```python
from build123d import *

# Parameters (mm, degrees)
BOSS_EXTRUDE2_DEPTH = 3
SKETCH2_W           = 44
SKETCH2_H           = 70
BOSS_EXTRUDE3_DEPTH = 10
BOSS_EXTRUDE4_DEPTH = 3
CUT_EXTRUDE1_REACH  = 103.047
SKETCH7_R           = 2.5


with BuildPart() as part:
    # Sketch1 → Boss-Extrude2 (new body)
    with BuildSketch(Plane.XY):
        with BuildLine():
            Line((-11.286595542, 0), (32.713404458, 0))
            Line((32.713404458, 0), (32.713404458, 49))
            Line((32.713404458, 49), (34.849610431, 49))
            Line((34.849610431, 49), (34.849610431, 64))
            Line((34.849610431, 64), (24.849610431, 64))
            Line((24.849610431, 64), (19.349610431, 45.378267854))
            Line((19.349610431, 45.378267854), (19.349610431, 40.378267854))
            ThreePointArc((19.349610431, 40.378267854), (9.849610431, 30.878267854), (0.349610431, 40.378267854))
            Line((0.349610431, 40.378267854), (0.349610431, 45.378267854))
            Line((0.349610431, 45.378267854), (-3.422801515, 64))
            Line((-3.422801515, 64), (-13.422801515, 64))
            Line((-13.422801515, 64), (-13.422801515, 49))
            Line((-13.422801515, 49), (-11.286595542, 49))
            Line((-11.286595542, 49), (-11.286595542, 0))
        make_face()
    extrude(amount=BOSS_EXTRUDE2_DEPTH)

    # Sketch2 → Boss-Extrude3 (add)
    with BuildSketch(Plane(origin=(0, 0, 0), x_dir=(1, 0, 0), z_dir=(0, 1, 0))):
        with Locations((10.713404458, 35)):
            Rectangle(SKETCH2_W, SKETCH2_H)
    extrude(amount=BOSS_EXTRUDE3_DEPTH)

    # Sketch4 → Boss-Extrude4 (add)
    with BuildSketch(Plane.XY.offset(-70)):
        with BuildLine():
            Line((34.849610431, 64), (24.849610431, 64))
            Line((24.849610431, 64), (19.349610431, 45.378267854))
            Line((19.349610431, 45.378267854), (19.349610431, 40.378267854))
            ThreePointArc((19.349610431, 40.378267854), (9.849610431, 30.878267854), (0.349610431, 40.378267854))
            Line((0.349610431, 40.378267854), (0.349610431, 45.378267854))
            Line((0.349610431, 45.378267854), (-3.422801515, 64))
            Line((-3.422801515, 64), (-13.422801515, 64))
            Line((-13.422801515, 64), (-13.422801515, 49))
            Line((-13.422801515, 49), (-11.286595542, 49))
            Line((-11.286595542, 49), (-11.286595542, 0))
            Line((-11.286595542, 0), (32.713404458, 0))
            Line((32.713404458, 0), (32.713404458, 49))
            Line((32.713404458, 49), (34.849610431, 49))
            Line((34.849610431, 49), (34.849610431, 64))
        make_face()
    extrude(amount=BOSS_EXTRUDE4_DEPTH)

    # Sketch7 → Cut-Extrude1 (cut, up to next)
    with BuildSketch(Plane(origin=(0, 0, 0), x_dir=(1, 0, 0), z_dir=(0, 1, 0)), mode=Mode.PRIVATE) as cut_extrude1_sk1:
        with Locations(Location((10.713404458, 48.5, 0), (0, 0, 270))):
            Circle(SKETCH7_R)
    cut_extrude1_tool1 = extrude(cut_extrude1_sk1.sketch, amount=CUT_EXTRUDE1_REACH, mode=Mode.PRIVATE) & part.part
    # Sketch7 → Cut-Extrude1 (cut, up to next)
    with BuildSketch(Plane(origin=(0, 0, 0), x_dir=(1, 0, 0), z_dir=(0, 1, 0)), mode=Mode.PRIVATE) as cut_extrude1_sk2:
        with Locations(Location((10.713404458, 18.5, 0), (0, 0, 270))):
            Circle(SKETCH7_R)
    cut_extrude1_tool2 = extrude(cut_extrude1_sk2.sketch, amount=CUT_EXTRUDE1_REACH, mode=Mode.PRIVATE) & part.part
    add(cut_extrude1_tool1.solids().sort_by_distance((10.713404, 0, -48.5))[0], mode=Mode.SUBTRACT)
    add(cut_extrude1_tool2.solids().sort_by_distance((10.713404, 0, -18.5))[0], mode=Mode.SUBTRACT)


solid = part.part
```
The model under review builds one solid part; all positions refer to its coordinate system, in mm. A direction names the side the tool comes from. Round coordinates to 2 decimals unless told otherwise and drop trailing zeros. Loops run counter-clockwise (first coordinate to the right, second up) from the corner with the lowest first, then second, coordinate; pieces in that order, holes last. Notation, with made-up numbers: (-21.75, 1.25) -> (-5.75, 1.25) arc R18 cw to (-5.75, 22.25) -> close; hole circle Ø4 at (36.25, -5.5). An arc over 180 degrees is marked (long way). Answer in a Markdown table with one row per item.
1) Consider section D-D, the plane x = 1.5. Write out the cut boundary in (y, z).
Taken from the geometry:
| item | result |
|---|---|
| outline | (0, -70) -> (35.85, -70) -> (35.85, -67) -> (10, -67) -> (10, 0) -> (35.85, 0) -> (35.85, 3) -> (0, 3) -> close |
2) For pin 1 Ø2.5 at (y, z) = (43, 1.5) entering from +X; pin 2 Ø1.1 at (x, z) = (34, 2) entering from -Y; pin 3 Ø13 at (x, z) = (-0.5, -33.5) entering from +Y; pin 4 Ø6 at (x, z) = (30, -53) entering from -Y, all flat-tipped, find the tip position at first contact; note any pin that passes through.
Taken from the geometry:
| item | result |
|---|---|
| pin 1 | stops at x = 32.71 |
| pin 2 | stops at y = 49 |
| pin 3 | stops at y = 10 |
| pin 4 | stops at y = 0 |
3) Draft analysis for pull direction X (two halves, no side actions). For faces 1 (the flat face through (0.35, 43, 1)), 2 (the flat face through (-11.287, 8, -26)), 3 (the flat face through (10, 0, -34)), 4 (the cylindrical face through (9.76, 4.93, -46.19)), state which applies: pulls with the +X half, pulls with the -X half, needs draft (parallel to the pull), parting line crosses it, or undercut.
Taken from the geometry:
| item | result |
|---|---|
| face 1 | undercut |
| face 2 | pulls with the -X half |
| face 3 | needs draft |
| face 4 | undercut |
4) Tool access review of faces 5 (the flat face through (10, 10, -34)), 6 (the flat face through (-12, 49, -69)), 7 (the flat face through (34, 49, 1)), 8 (the flat face through (-1.51, 54.56, 1.48)): name each direction out of +Z, -Z, +X, -X, +Y, -Y from which nothing blocks a thin tool from reaching the whole face with its end or side.
Taken from the geometry:
| item | result |
|---|---|
| face 5 | +X, -X, +Y |
| face 6 | +Z, -Z, -X, -Y |
| face 7 | +Z, -Z, +X, -Y |
| face 8 | +Z, -Z, +Y |
5) Wall thickness on line 1 along Z through (x, y) = (11, 30.5); line 2 along X through (y, z) = (7.5, -48.5); line 3 along Y through (x, z) = (14.5, -13): over which ranges is each line inside the solid? List them lowest first.
Taken from the geometry:
| item | result |
|---|---|
| line 1 | z = -70 to -67, 0 to 3 |
| line 2 | x = -11.29 to 8.21, 13.21 to 32.71 |
| line 3 | y = 0 to 10 |
6) Consider section B-B, the plane z = -48.5. Write out the cut boundary in (x, y).
Taken from the geometry:
| item | result |
|---|---|
| outline | (-11.29, 0) -> (8.21, 0) -> (8.21, 10) -> (-11.29, 10) -> close; (13.21, 0) -> (32.71, 0) -> (32.71, 10) -> (13.21, 10) -> close |
7) Consider section C-C, the plane y = 42. Write out the cut boundary in (x, z).
Taken from the geometry:
| item | result |
|---|---|
| outline | (-11.29, -70) -> (0.35, -70) -> (0.35, -67) -> (-11.29, -67) -> close; (-11.29, 0) -> (0.35, 0) -> (0.35, 3) -> (-11.29, 3) -> close; (19.35, -70) -> (32.71, -70) -> (32.71, -67) -> (19.35, -67) -> close; (19.35, 0) -> (32.71, 0) -> (32.71, 3) -> (19.35, 3) -> close |
8) Consider section A-A, the plane y = 25. Write out the cut boundary in (x, z).
Taken from the geometry:
| item | result |
|---|---|
| outline | (-11.29, -70) -> (32.71, -70) -> (32.71, -67) -> (-11.29, -67) -> close; (-11.29, 0) -> (32.71, 0) -> (32.71, 3) -> (-11.29, 3) -> close |
